Read the model definition and answer for the solid it produces. Units are mm, in the model's axes. A direction names the side the tool comes from. Round coordinates to 2 decimals unless told otherwise and drop trailing zeros. Order: outer loops, then holes, each group sorted by start corner. A loop starts at its lowest first (then second) coordinate and runs counter-clockwise, first axis right, second up. Notation, with made-up numbers: M 13,72.5 L 60,72.5 A16 cw 60,95.5 Z; hole C 51,-26 d3. An arc over 180 degrees is marked long. Use one line per item in the form item = value. Start each with the question number.
from build123d import *

# Parameters (mm, degrees)
F0_R     = 1
F0_R_2   = 1.5
F0_R_3   = 2
F1_DEPTH = 6
F3_DEPTH = 8
F5_DEPTH = 25
F7_DEPTH = 25
F9_DEPTH = 13


# Not quite as in the source:
# - a feature names something its author has since deleted; it is built from what else it names


with BuildPart() as f1:
    # F0 (on Top) → F1 (new body)
    with BuildSketch(Plane.XY):
        with BuildLine():
            Line((-42.1966487169, -12.8954221606), (-42.1966487169, -25.8954221606))
            Line((-42.1966487169, -25.8954221606), (17.9292613268, -25.8954221606))
            Line((17.9292613268, -25.8954221606), (47.9292613268, -25.8954221606))
            Line((47.9292613268, -25.8954221606), (47.9292613268, -12.8954221606))
            Line((47.9292613268, -12.8954221606), (20.3033512831, -12.8954221606))
            ThreePointArc((20.3033512831, -12.8954221606), (17.8033512831, -15.3954221606), (15.3033512831, -12.8954221606))
            Line((15.3033512831, -12.8954221606), (4.8663063049, -12.8954221606))
            ThreePointArc((4.8663063049, -12.8954221606), (2.8663063049, -14.8954221606), (0.8663063049, -12.8954221606))
            Line((0.8663063049, -12.8954221606), (-10.6966487169, -12.8954221606))
            ThreePointArc((-10.6966487169, -12.8954221606), (-12.1966487169, -14.3954221606), (-13.6966487169, -12.8954221606))
            Line((-13.6966487169, -12.8954221606), (-26.1966487169, -12.8954221606))
            ThreePointArc((-26.1966487169, -12.8954221606), (-27.1966487169, -13.8954221606), (-28.1966487169, -12.8954221606))
            Line((-28.1966487169, -12.8954221606), (-42.1966487169, -12.8954221606))
        make_face()
        with Locations((-27.0707386732, -19.3954221606)):
            Circle(F0_R, mode=Mode.SUBTRACT)
        with Locations((-12.0707386732, -19.3954221606)):
            Circle(F0_R_2, mode=Mode.SUBTRACT)
        with Locations((2.9292613268, -19.3954221606)):
            Circle(F0_R_3, mode=Mode.SUBTRACT)
        with BuildLine():
            ThreePointArc((20.4292613268, -19.3954221606), (19.6970282798, -21.1631891136), (17.9292613268, -21.8954221606))
            ThreePointArc((17.9292613268, -21.8954221606), (16.1614943738, -17.6276552077), (20.4292613268, -19.3954221606))
        make_face(mode=Mode.SUBTRACT)
        with BuildLine():
            ThreePointArc((-102.1092408178, -21.9157785711), (-100.9305134828, -24.7310372299), (-98.109292616, -25.8954221606))
            Line((-98.109292616, -25.8954221606), (-42.1966487169, -25.8954221606))
            Line((-42.1966487169, -25.8954221606), (-42.1966487169, -12.8954221606))
            Line((-42.1966487169, -12.8954221606), (-98.1347384587, -12.8954221606))
            ThreePointArc((-98.1347384587, -12.8954221606), (-100.9703535279, -14.0742012939), (-102.1346866604, -16.9157785711))
            Line((-102.1346866604, -16.9157785711), (-102.1092408178, -21.9157785711))
        make_face()
    extrude(amount=F1_DEPTH)

    # F2 (on face) → F3 (join)
    with BuildSketch(Plane(origin=(0, 0, 0), x_dir=(1, 0, 0), z_dir=(0, 0, -1))):
        with BuildLine():
            Line((47.9292613268, 25.8954221606), (47.9292613268, 12.8954221606))
            Line((47.9292613268, 12.8954221606), (67.9292613268, 10.8954221606))
            Line((67.9292613268, 10.8954221606), (67.9292613268, 15.8954221606))
            Line((67.9292613268, 15.8954221606), (63.9292613268, 15.8954221606))
            ThreePointArc((63.9292613268, 15.8954221606), (60.4292613268, 19.3954221606), (63.9292613268, 22.8954221606))
            Line((63.9292613268, 22.8954221606), (67.9292613268, 22.8954221606))
            Line((67.9292613268, 22.8954221606), (67.9292613268, 27.8954221606))
            Line((67.9292613268, 27.8954221606), (47.9292613268, 25.8954221606))
        make_face()
    extrude(amount=-F3_DEPTH)

    # F4 (on face) → F5 (cut)
    with BuildSketch(Plane(origin=(-2.0893560424, -20.8935604237, 0), x_dir=(0.9950371902, -0.099503719, 0), z_dir=(-0.099503719, -0.9950371902, 0))):
        with BuildLine():
            Line((47.7105565369, 6), (50.2680883301, 6))
            Line((50.2680883301, 6), (50.2680883301, 8))
            Line((50.2680883301, 8), (70.3678395723, 8))
            add(Edge.make_bspline(
                [(70.3678395723, 8), (72.5767643682, 9.8820103785), (72.4269967916, 13.5723014467), (72.296127677, 17.0164462179)],
                knots=[0.596790788, 0.596790788, 0.596790788, 0.596790788, 1, 1, 1, 1], degree=3))
            add(Edge.make_bspline(
                [(70.3678395723, 5.5720340461), (72.8712183365, 8.3489220533), (72.5836730067, 12.6826841356), (72.296127677, 17.0164462179)],
                knots=[0.5727584581, 0.5727584581, 0.5727584581, 0.5727584581, 1, 1, 1, 1], degree=3))
            Line((70.3678395723, 5.5720340461), (70.3678395723, 0))
            Line((70.3678395723, 0), (50.2680883301, 0))
            Line((50.2680883301, 0), (50.2680883301, -3.928697668))
            Line((50.2680883301, -3.928697668), (74.866913259, -3.928697668))
            Line((74.866913259, -3.928697668), (74.866913259, 21.5322930813))
            Line((74.866913259, 21.5322930813), (50.2680883301, 21.5322930813))
            Line((50.2680883301, 21.5322930813), (47.7105565369, 21.5322930813))
            Line((47.7105565369, 21.5322930813), (47.7105565369, 6))
        make_face()
        with BuildLine():
            Line((50.2680883301, 8), (50.2680883301, 6))
            add(Edge.make_bspline(
                [(50.2680883301, 6), (58.6617788579, 6.3902694532), (67.098405416, 5.2144325486), (70.3678395723, 8)],
                knots=[0, 0, 0, 0, 0.596790788, 0.596790788, 0.596790788, 0.596790788], degree=3))
            Line((70.3678395723, 8), (50.2680883301, 8))
        make_face()
        with BuildLine():
            add(Edge.make_bspline(
                [(50.2680883301, 0), (58.6399537153, 0.9246740387), (67.0118191006, 1.8493480774), (70.3678395723, 5.5720340461)],
                knots=[0, 0, 0, 0, 0.5727584581, 0.5727584581, 0.5727584581, 0.5727584581], degree=3))
            Line((50.2680883301, 0), (70.3678395723, 0))
            Line((70.3678395723, 0), (70.3678395723, 5.5720340461))
        make_face()
    extrude(amount=-F5_DEPTH, mode=Mode.SUBTRACT)

    # F6 (on face) → F7 (cut)
    with BuildSketch(Plane.XZ.offset(25.8954221606)):
        Polygon((-103.6658883095, 0), (-101.9829884171, 0.653559342), (-72.109292616, 6), (-72.109292616, 8.9457267895), (-103.4941226244, 6.6766636446), align=None)
    extrude(amount=-F7_DEPTH, mode=Mode.SUBTRACT)

    # F8 (on face) → F9 (join)
    with BuildSketch(Plane.XZ.offset(25.8954221606)):
        Polygon((-67.109292616, 7), (-69.109292616, 6), (-67.109292616, 6), (-56.109292616, 6), (-59.109292616, 8), (-64.109292616, 8), (-66.109292616, 7), align=None)
    extrude(amount=-F9_DEPTH)


solid = f1.part
Item 1: For a pull along Y with two mould halves and no side action, classify faces 4 (the cylindrical face through (-13.176, -18.382, 2.958)), 5 (the flat face through (-4, -19, 6)), 6 (the flat face through (55.847, -26.687, 3.944)) as pulls with the +Y half, pulls with the -Y half, needs draft (parallel to the pull), parting line crosses it, or undercut.
Item 2: Section A-A (x = -22.5) is taken. Write down the section's boundary in (y, z), and give its area (3 significant figures).
Item 3: Find the intervals of material crossed by L1, parallel to Y at x = -63.5, z = 3.25; L2, parallel to Z at x = -27, y = -24.75; L3, parallel to Z at x = -90, y = -19.5, in increasing order. Write a range as [from, to].
Item 4: A tool of negligible diameter and unlimited length cuts with its end or side. For faces 1 (the flat face through (66, -22.895, 5)), 2 (the flat face through (-20, -12.895, 3)), 3 (the flat face through (-71, -19, 6)), from which of +Z, -Z, +X, -X, +Y, -Y can it reach the whole face along a straight path? Write none if from no direction.
Item 5: Given P1, Ø2.5, axis at x = -48.5, z = 5.5, coming from the +Y side; P2, Ø10, axis at x = 16.5, y = -26, coming from the +Z side; P3, Ø3, axis at x = -70.5, z = 4.5, coming from the -Y side, each flat-ended and moving along its own axis, determine where each tip first touches the part or whether it passes through.
Item 6: Section B-B (x = -79) is taken. Write down the section's boundary in (y, z).
The answers:
q1.face_4 = undercut
q1.face_5 = needs draft
q1.face_6 = pulls with the -Y half
q2.outline = M -25.9,0 L -12.9,0 L -12.9,6 L -25.9,6 Z
q2.area = 78.0 mm²
q3.L1 = [-25.9, -12.9]
q3.L2 = [0, 6]
q3.L3 = [0, 2.8]
q4.face_1 = +Z, -Z, +X
q4.face_2 = +Z, -Z, -X, +Y
q4.face_3 = +Z, -X, +Y, -Y
q5.P1 = -12.9
q5.P2 = 6
q5.P3 = -25.9
q6.outline = M -25.9,0 L -12.9,0 L -12.9,4.77 L -25.9,4.77 Z
